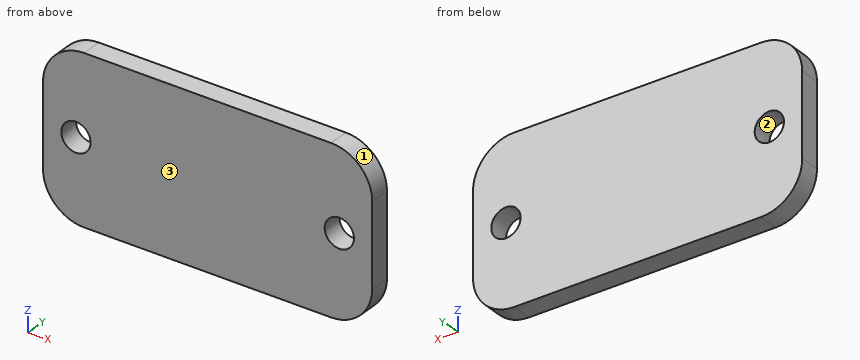
```python
from build123d import *

# Parameters (mm, degrees)
SKETCH1_W           = 25.4
SKETCH1_H           = 12.7
BOSS_EXTRUDE1_DEPTH = 1.5875
FILLET1_R           = 3.175
SKETCH2_R           = 1.1303
CUT_EXTRUDE1_DEPTH  = 29.442400677


with BuildPart() as part:
    # Sketch1 → Boss-Extrude1 (new body)
    with BuildSketch(Plane(origin=(0, 0, 0), x_dir=(1, 0, 0), z_dir=(0, 1, 0))):
        with Locations((12.7, 6.35)):
            Rectangle(SKETCH1_W, SKETCH1_H)
    extrude(amount=BOSS_EXTRUDE1_DEPTH)

    # Fillet1
    fillet1_edges = [part.edges().sort_by_distance(p)[0] for p in [
        (0, 0.79375, -12.7),
        (25.4, 0.79375, -12.7),
        (25.4, 0.79375, 0),
        (0, 0.79375, 0),
    ]]
    fillet(fillet1_edges, radius=FILLET1_R)

    # Sketch2 → Cut-Extrude1 (cut, through all)
    with BuildSketch(Plane(origin=(0, 1.5875, 0), x_dir=(1, 0, 0), z_dir=(0, 1, 0))):
        with Locations(Location((2.54, 6.35, 0), (0, 0, 270))):
            Circle(SKETCH2_R)
        with Locations(Location((22.86, 6.35, 0), (0, 0, 90))):
            Circle(SKETCH2_R)
    extrude(amount=-CUT_EXTRUDE1_DEPTH, mode=Mode.SUBTRACT)


solid = part.part
```
The listing builds one solid part. Answer for the finished solid, in the listing's coordinates (mm). Face numbers are marked on the shaded views. Coordinates: 2 decimals unless noted, no trailing zeros. Loops run counter-clockwise (first coordinate to the right, second up) from the corner with the lowest first, then second, coordinate; pieces in that order, holes last. Notation, with made-up numbers: M 84,-24 L 109,-24 A22 ccw 109,-13 Z; hole C 77,40.25 d3. An arc over 180 degrees is marked long. Answer as CSV lines item,"result". Start each with the question number.
(1) Given pin 1 (1.4 mm diameter, centred on x = 2.54, z = -6.35, fed in from -Y), flat-ended and moving along its own axis, determine where the tip first touches the part or whether it passes through.
(2) The part is cut by section B-B (y = 0.55). Give the vertices of the cut face in (x, z) (3 decimals).
(3) Find the intervals of material crossed by L1, parallel to X at y = 1.05, z = -6.35; L2, parallel to X at y = 0.6, z = -5.5; L3, parallel to Z at x = 22.86, y = 1.25, in increasing order. Write a range as [from, to].
(4) The part is cut by section C-C (x = 22.86). Give the vertices of the cut face in (y, z), and give its area (3 significant figures).
(5) The part is cut by section A-A (z = -6.35). Give the vertices of the cut face in (x, y).
(6) The part is cut by section D-D (z = -1.75). Give the vertices of the cut face in (x, y), and give its area (3 significant figures).
(7) The mould has two halves that part along Z. Classify the marked faces 1, 2 and 3: pulls with the +Z half, pulls with the -Z half, needs draft (parallel to the pull), parting line crosses it, or undercut.
Determined:
1,pin 1,"through"
2,outline,"M 0,-9.525 A3.175 ccw 3.175,-12.7 L 22.225,-12.7 A3.175 ccw 25.4,-9.525 L 25.4,-3.175 A3.175 ccw 22.225,0 L 3.175,0 A3.175 ccw 0,-3.175 Z; hole C 2.54,-6.35 d2.261; hole C 22.86,-6.35 d2.261"
3,L1,"[0, 1.41], [3.67, 21.73], [23.99, 25.4]"
3,L2,"[0, 1.79], [3.29, 22.11], [23.61, 25.4]"
3,L3,"[-12.64, -7.48], [-5.22, -0.06]"
4,outline,"M 0,-12.64 L 1.59,-12.64 L 1.59,-7.48 L 0,-7.48 Z; M 0,-5.22 L 1.59,-5.22 L 1.59,-0.06 L 0,-0.06 Z"
4,area,"16.4 mm2"
5,outline,"M 0,0 L 1.41,0 L 1.41,1.59 L 0,1.59 Z; M 3.67,0 L 21.73,0 L 21.73,1.59 L 3.67,1.59 Z; M 23.99,0 L 25.4,0 L 25.4,1.59 L 23.99,1.59 Z"
6,outline,"M 0.34,0 L 25.06,0 L 25.06,1.59 L 0.34,1.59 Z"
6,area,"39.3 mm2"
7,face 1,"pulls with the +Z half"
7,face 2,"undercut"
7,face 3,"needs draft"
